Design review of the part built by this model. Coordinates are the model's own, in mm. Face numbers are marked on the shaded views. A direction names the side the tool comes from. Give positions to 0.01 mm unless a question says otherwise; leave off trailing zeros. Loops run counter-clockwise (first coordinate to the right, second up) from the corner with the lowest first, then second, coordinate; pieces in that order, holes last. Notation, with made-up numbers: (20, 86) - (31, 86) arc R15 cw to (31, 109) - close; hole circle Ø9 at (62.5, 8.25). An arc over 180 degrees is marked (long way). One line per item, written item: value. Start each with the question number.
```python
from build123d import *

# Parameters (mm, degrees)
SKETCH008_R             = 1.75
PAD001_DEPTH            = 21
SKETCH009_W             = 5.5
SKETCH009_H             = 2.4
POCKET003_DEPTH         = 8
SKETCH010_R             = 3.1
POCKET004_DEPTH         = 3
SKETCH014_W             = 1.5
SKETCH014_H             = 2
SKETCH014_W_2           = 2.5
SKETCH014_H_2           = 1.5
POCKET005_DEPTH         = 21.001
BODY002_ROLL_ANGLE      = 180
BODY002_PLACEMENT_ANGLE = 90
SKETCH_R                = 1.75
PAD_DEPTH               = 21
SKETCH002_W             = 5.5
SKETCH002_H             = 2.4
POCKET_DEPTH            = 8
SKETCH003_R             = 3.1
POCKET001_DEPTH         = 3
SKETCH007_W             = 1.5
SKETCH007_H             = 2
SKETCH007_W_2           = 2.5
SKETCH007_H_2           = 1.5
POCKET002_DEPTH         = 21.001


with BuildPart() as body002:
    # Sketch008 → Pad001 (new body)
    with BuildSketch(Plane.YZ):
        with BuildLine():
            Line((-5, 8), (-5, 10))
            Line((-5, 10), (5, 10))
            Line((5, 10), (5, 8))
            ThreePointArc((5, 8), (3.556624, 5.5), (5, 3))
            Line((5, 3), (5, 0))
            Line((5, 0), (2.5, 0))
            ThreePointArc((2.5, 0), (0, 1.443376), (-2.5, 0))
            Line((-2.5, 0), (-5, 0))
            Line((-5, 0), (-5, 3))
            ThreePointArc((-5, 3), (-3.556624, 5.5), (-5, 8))
        make_face()
        with Locations((0, 5)):
            Circle(SKETCH008_R, mode=Mode.SUBTRACT)
    extrude(amount=PAD001_DEPTH)

    # Sketch009 → Pocket003 (cut)
    with BuildSketch(Plane(origin=(0, 0, 10), x_dir=(0, -1, 0), z_dir=(0, 0, 1))):
        with Locations((0, 5.7)):
            Rectangle(SKETCH009_W, SKETCH009_H)
        with Locations((0, 18.2)):
            Rectangle(SKETCH009_W, SKETCH009_H)
    extrude(amount=-POCKET003_DEPTH, mode=Mode.SUBTRACT)

    # Sketch010 (on Face4 of Pocket003) → Pocket004 (cut)
    with BuildSketch(Plane(origin=(0, 0, 0), x_dir=(0, 1, 0), z_dir=(-1, 0, 0))):
        with Locations((0, -5)):
            Circle(SKETCH010_R)
    extrude(amount=-POCKET004_DEPTH, mode=Mode.SUBTRACT)

    # Sketch014 (on Face4 of Pocket004) → Pocket005 (cut, through all)
    with BuildSketch(Plane(origin=(0, 0, 0), x_dir=(0, 1, 0), z_dir=(-1, 0, 0))):
        with Locations((-3.5, -1.75)):
            Rectangle(SKETCH014_W, SKETCH014_H)
        with Locations((3.5, -1.75)):
            Rectangle(SKETCH014_W, SKETCH014_H)
        with Locations((-2.75, -8.75)):
            Rectangle(SKETCH014_W_2, SKETCH014_H_2)
        with Locations((2.75, -8.75)):
            Rectangle(SKETCH014_W_2, SKETCH014_H_2)
    extrude(amount=-POCKET005_DEPTH, mode=Mode.SUBTRACT)


with BuildPart() as body002_1:
    # Body002 roll: moved
    add(body002.part.rotate(Axis((0, 0, 0), (1, 0, 0)), BODY002_ROLL_ANGLE))


with BuildPart() as body002_2:
    # Body002 placement: moved
    add(body002_1.part.moved(Location((12, -12, 19))).rotate(Axis((12, -12, 19), (0, 0, 1)), BODY002_PLACEMENT_ANGLE))


with BuildPart() as fusion:
    # Sketch → Pad (new body)
    with BuildSketch(Plane.YZ):
        with BuildLine():
            Line((-5, 8), (-5, 10))
            Line((-5, 10), (5, 10))
            Line((5, 10), (5, 8))
            ThreePointArc((5, 8), (3.556624, 5.5), (5, 3))
            Line((5, 3), (5, 0))
            Line((5, 0), (2.5, 0))
            ThreePointArc((2.5, 0), (0, 1.443376), (-2.5, 0))
            Line((-2.5, 0), (-5, 0))
            Line((-5, 0), (-5, 3))
            ThreePointArc((-5, 3), (-3.556624, 5.5), (-5, 8))
        make_face()
        with Locations((0, 5)):
            Circle(SKETCH_R, mode=Mode.SUBTRACT)
    extrude(amount=PAD_DEPTH)

    # Sketch002 → Pocket (cut)
    with BuildSketch(Plane(origin=(0, 0, 10), x_dir=(0, -1, 0), z_dir=(0, 0, 1))):
        with Locations((0, 5.7)):
            Rectangle(SKETCH002_W, SKETCH002_H)
        with Locations((0, 18.2)):
            Rectangle(SKETCH002_W, SKETCH002_H)
    extrude(amount=-POCKET_DEPTH, mode=Mode.SUBTRACT)

    # Sketch003 (on Face4 of Pocket) → Pocket001 (cut)
    with BuildSketch(Plane(origin=(0, 0, 0), x_dir=(0, 1, 0), z_dir=(-1, 0, 0))):
        with Locations((0, -5)):
            Circle(SKETCH003_R)
    extrude(amount=-POCKET001_DEPTH, mode=Mode.SUBTRACT)

    # Sketch007 (on Face4 of Pocket001) → Pocket002 (cut, through all)
    with BuildSketch(Plane(origin=(0, 0, 0), x_dir=(0, 1, 0), z_dir=(-1, 0, 0))):
        with Locations((-3.5, -1.75)):
            Rectangle(SKETCH007_W, SKETCH007_H)
        with Locations((3.5, -1.75)):
            Rectangle(SKETCH007_W, SKETCH007_H)
        with Locations((-2.75, -8.75)):
            Rectangle(SKETCH007_W_2, SKETCH007_H_2)
        with Locations((2.75, -8.75)):
            Rectangle(SKETCH007_W_2, SKETCH007_H_2)
    extrude(amount=-POCKET002_DEPTH, mode=Mode.SUBTRACT)

    # Fusion: union Body002
    add(body002_2.part)


solid = fusion.part
```
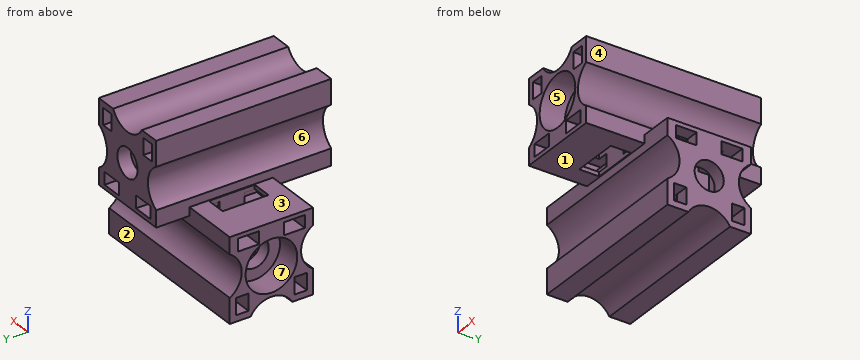
(1) Machinability: for the marked faces 1, 2 and 3, which of the approach directions +Z, -Z, +X, -X, +Y, -Y give a long, thin tool a straight path to every point of the face, cutting with its end or side? Answer none if there is none.
(2) Take a section at B-B on z = 5. State the section outline as (x, y) points.
(3) For pin 1 Ø6 at (y, z) = (-8.5, 13) entering from -X; pin 2 Ø1.9 at (x, y) = (12.5, 6.5) entering from -Z; pin 3 Ø1 at (y, z) = (-2.5, 17.5) entering from +X, all flat-tipped, find the tip position at first contact; note any pin that passes through.
(4) To check wall thickness, follow L1, parallel to X at y = -1.75, z = 2.5; L2, parallel to Z at x = 3.45, y = 0; L3, parallel to Z at x = 1.45, y = 0. State the ranges of each line that lie inside material, in increasing order. Write a range as from..to.
(5) Take a section at A-A on y = 0. State how many separate pieces and enclosed holes the cut face has, and give its area (3 significant figures).
(6) Draft analysis for pull direction X (two halves, no side actions). For the marked faces 4, 5, 6 and 7, state which applies: pulls with the +X half, pulls with the -X half, needs draft (parallel to the pull), parting line crosses it, or undercut.
Here are the results:
1. face 1: -Z, +X, -X, -Y
1. face 2: -Z, +X, -X, +Y
1. face 3: +Z, -X, +Y, -Y
2. outline: (0, -3.6) - (21, -3.6) - (21, -1.75) - (19.4, -1.75) - (19.4, -2.75) - (17, -2.75) - (17, -1.75) - (6.9, -1.75) - (6.9, -2.75) - (4.5, -2.75) - (4.5, -1.75) - (3, -1.75) - (3, -3.1) - (0, -3.1) - close; (0, 3.1) - (3, 3.1) - (3, 1.75) - (4.5, 1.75) - (4.5, 2.75) - (6.9, 2.75) - (6.9, 1.75) - (17, 1.75) - (17, 2.75) - (19.4, 2.75) - (19.4, 1.75) - (21, 1.75) - (21, 3.6) - (0, 3.6) - close
3. pin 1: x = 7
3. pin 2: z = 9
3. pin 3: x = 17
4. L1: 3..4.5, 6.9..17, 19.4..21
4. L2: 1.44..3.25, 6.75..10
4. L3: 1.44..1.9, 8.1..10
5. separate pieces: 4
5. enclosed holes: 5
5. area: 131 mm²
6. face 4: pulls with the +X half
6. face 5: undercut
6. face 6: pulls with the -X half
6. face 7: needs draft
